Here's how the part is built. I have some questions about the finished solid (model axes, mm). A direction names the side the tool comes from. Round coordinates to 2 decimals unless told otherwise and drop trailing zeros. Order: outer loops, then holes, each group sorted by start corner. A loop starts at its lowest first (then second) coordinate and runs counter-clockwise, first axis right, second up. Notation, with made-up numbers: (89, 76.5) -> (101, 76.5) arc R34 ccw to (101, 107.5) -> close; hole circle Ø10 at (-9, -39.75). An arc over 180 degrees is marked (long way). One line per item, written item: value.
```python
from build123d import *

# Parameters (mm, degrees)
F2_DEPTH  = 9.525
F4_DEPTH  = 304.8
F6_DEPTH  = 63.5
F8_W      = 63.5
F8_H      = 63.5
F8_W_2    = 50.8
F8_H_2    = 50.8
F9_DEPTH  = 228.6
F11_DEPTH = 128.262011


with BuildPart() as f2:
    # F1 (on face) → F2 (new body)
    with BuildSketch(Plane.XY):
        Polygon((-48.886011, -84.673055), (144.136011, -84.673055), (95.25, 0), (0, 0), align=None)
    extrude(amount=F2_DEPTH)

    # F3 (on face) → F4 (join)
    with BuildSketch(Plane.XY.offset(9.525)):
        Polygon((79.375, -10.586528), (47.625, -10.586528), (47.625, -16.936528), (73.025, -16.936528), (73.025, -67.736528), (47.625, -67.736528), (47.625, -74.086528), (79.375, -74.086528), align=None)
        Polygon((47.625, -16.936528), (47.625, -10.586528), (15.875, -10.586528), (15.875, -74.086528), (47.625, -74.086528), (47.625, -67.736528), (22.225, -67.736528), (22.225, -16.936528), align=None)
    extrude(amount=F4_DEPTH)

    # F5 (on face) → F6 (cut)
    with BuildSketch(Plane.YZ.offset(79.375)):
        Polygon((-10.586528, 314.325), (-74.086528, 314.325), (-10.586528, 250.825), align=None)
    extrude(amount=-F6_DEPTH, mode=Mode.SUBTRACT)

    # F8 (on face) → F9 (join)
    with BuildSketch(Plane.XZ.offset(74.086528)):
        with Locations((47.625, 282.575)):
            Rectangle(F8_W, F8_H)
        with Locations((47.625, 282.575)):
            Rectangle(F8_W_2, F8_H_2, mode=Mode.SUBTRACT)
    extrude(amount=-F9_DEPTH)

    # F10 (on face) → F11 (cut, through all)
    with BuildSketch(Plane.YZ.offset(79.375)):
        Polygon((91.013472, 314.325), (154.513472, 250.825), (154.513472, 314.325), align=None)
    extrude(amount=-F11_DEPTH, mode=Mode.SUBTRACT)


solid = f2.part
```
Q1. I want a section at B-B on z = 41. Write out the boundary of the cut face in (x, y) (3 decimals).
Answers:
outline: (15.875, -74.087) -> (79.375, -74.087) -> (79.375, -10.587) -> (15.875, -10.587) -> close; hole (22.225, -67.737) -> (73.025, -67.737) -> (73.025, -16.937) -> (22.225, -16.937) -> close
Q2. If we mould it in two halves opening along X, with no side actions, what happens to faces 1 (the face through (79.375, -12, 194)), 2 (the face through (47, -42, 9.525)), 3 (the face through (47, 7, 314.325))? For each: pulls with the +X half, pulls with the -X half, needs draft (parallel to the pull), parting line crosses it, or undercut.
Answers:
face 1: pulls with the +X half
face 2: undercut
face 3: needs draft
Q3. I want a section at A-A on y = 72. Write out the boundary of the cut face in (x, z) (3 decimals).
Answers:
outline: (15.875, 250.825) -> (79.375, 250.825) -> (79.375, 314.325) -> (15.875, 314.325) -> close; hole (22.225, 257.175) -> (73.025, 257.175) -> (73.025, 307.975) -> (22.225, 307.975) -> close
Q4. I want a section at C-C on x = 62.5. Write out the boundary of the cut face in (y, z) (3 decimals).
Answers:
outline: (-84.673, 0) -> (0, 0) -> (0, 9.525) -> (-10.587, 9.525) -> (-10.587, 250.825) -> (154.513, 250.825) -> (148.163, 257.175) -> (-67.737, 257.175) -> (-67.737, 307.975) -> (97.363, 307.975) -> (91.013, 314.325) -> (-74.087, 314.325) -> (-74.087, 9.525) -> (-84.673, 9.525) -> close; hole (-67.737, 9.525) -> (-16.937, 9.525) -> (-16.937, 250.825) -> (-67.737, 250.825) -> close
Q5. I want a section at D-D on y = -4. Write out the boundary of the cut face in (x, z) (3 decimals).
Answers:
outline: (-2.309, 0) -> (97.559, 0) -> (97.559, 9.525) -> (-2.309, 9.525) -> close; (15.875, 250.825) -> (79.375, 250.825) -> (79.375, 314.325) -> (15.875, 314.325) -> close; hole (22.225, 257.175) -> (73.025, 257.175) -> (73.025, 307.975) -> (22.225, 307.975) -> close
Q6. For P1, Ø1, axis at x = 43.5, z = 124.5, coming from the -Y side; P2, Ø10, axis at x = 14.5, y = 16.5, coming from the -Z side (3 decimals); P3, Ø5, axis at x = 77, z = 129.5, coming from the +Y side, each with a flat end and sliding along its axis, tell me the tip position at first contact or that it passes through.
Answers:
P1: y = -74.09
P2: z = 250.825
P3: y = -10.59
Q7. Which directions (+Z, -Z, +X, -X, +Y, -Y) give clear straight access to the entire face, cutting with the end or side of a thin tool? Please do faces 4 (the face through (48, 0, 5)), 5 (the face through (47, -16.937, 128)), 6 (the face through (22.225, 39, 282)), 7 (the face through (47, -74.087, 160)), 8 (the face through (15.875, -34, 194)).
Answers:
face 4: -Z, +X, -X, +Y
face 5: none
face 6: +Y
face 7: +Z, +X, -X, -Y
face 8: +Z, -X, +Y, -Y
Q8. I need wall thicknesses on line 1 along Z through (x, y) = (46, -54) (3 decimals); line 2 along Y through (x, z) = (27.5, 94); line 3 along X through (y, z) = (-49, 19) (3 decimals). Which ranges of each line are inside material? Lowest first, please.
Answers:
line 1: 0 to 9.525, 250.825 to 257.175, 307.975 to 314.325
line 2: -74.09 to -67.74, -16.94 to -10.59
line 3: 15.875 to 22.225, 73.025 to 79.375
